from build123d import *

# Parameters (mm, degrees)
F1_DEPTH = 250
F2_R     = 175
F3_DEPTH = 200


with BuildPart() as f1:
    # F0 (on Front) → F1 (new body)
    with BuildSketch(Plane.XZ):
        with BuildLine():
            Line((400, -800), (400, 0))
            ThreePointArc((400, 0), (0, 400), (-400, 0))
            Line((-400, 0), (-400, -800))
            Line((-400, -800), (-150, -800))
            Line((-150, -800), (-150, -606.184542))
            Line((-150, -606.184542), (150, -606.184542))
            Line((150, -606.184542), (150, -800))
            Line((150, -800), (400, -800))
        make_face()
    extrude(amount=F1_DEPTH)

    # F2 (on face) → F3 (join)
    with BuildSketch(Plane.XZ.offset(250)):
        Circle(F2_R)
    extrude(amount=F3_DEPTH)


solid = f1.part
For this review, take the finished solid that the model builds, in its own axes (mm). A direction names the side the tool comes from. Coordinates: 2 decimals unless noted, no trailing zeros. Order: outer loops, then holes, each group sorted by start corner. A loop starts at its lowest first (then second) coordinate and runs counter-clockwise, first axis right, second up. Notation, with made-up numbers: (56, 56) - (65, 56) arc R16 ccw to (65, 65) - close; hole circle Ø10 at (19, 54.5). An arc over 180 degrees is marked (long way). Answer as CSV lines item,"result". Start each with the question number.
1) Add section B-B (x = 0). State the section outline as (y, z) points, then the cut area to 3 significant figures.
2) Insertion check: P1, Ø2, axis at x = 281, y = -96.5, coming from the +Z side; P2, Ø6, axis at x = 112.5, y = -81.5, coming from the -Z side; P3, Ø3, axis at y = -111, z = 117, coming from the -X side. Each pin has a flat end and moves straight along its axis. Give the tip position at first contact, or say it passes through.
3) Add section A-A (y = -94.5). State the section outline as (x, z) points, then the cut area to 3 significant figures.
4) Add section C-C (z = -262.5). State the section outline as (x, y) points, then the cut area to 3 significant figures.
5) Machinability: for faces 1 (the flat face through (-2, -450, 2)), 2 (the flat face through (150, -123, -702)), 3 (the cylindrical face through (-128.982, -348.6, 118.273)), which of the approach directions +Z, -Z, +X, -X, +Y, -Y give a long, thin tool a straight path to every point of the face, cutting with its end or side? Answer none if there is none.
6) Draft analysis for pull direction X (two halves, no side actions). For faces 4 (the flat face through (400, -123, -406)), 5 (the flat face through (-2, -123, -606.185)), 6 (the cylindrical face through (8.796, -123.25, 399.903)), state which applies: +X half, -X half, draft (parallel to the pull), parting line (faces both ways), or undercut.
7) To check wall thickness, follow line 1 along X through (y, z) = (-34.5, -650.5); line 2 along Y through (x, z) = (-284, -90.5); line 3 along X through (y, z) = (-408.5, 9.5). State the ranges of each line that lie inside material, in increasing order. Write a range as [from, to].
8) Add section D-D (y = -280). State the section outline as (x, z) points, then the cut area to 3 significant figures.
Result:
1,outline,"(-450, -175) - (-250, -175) - (-250, -606.18) - (0, -606.18) - (0, 400) - (-250, 400) - (-250, 175) - (-450, 175) - close"
1,area,"322,000 mm^2"
2,P1,"z = 285.66"
2,P2,"z = -606.18"
2,P3,"x = -382.96"
3,outline,"(-400, -800) - (-150, -800) - (-150, -606.18) - (150, -606.18) - (150, -800) - (400, -800) - (400, 0) arc R400 ccw to (-400, 0) - close"
3,area,"833,000 mm^2"
4,outline,"(-400, -250) - (400, -250) - (400, 0) - (-400, 0) - close"
4,area,"200,000 mm^2"
5,face 1,"+Z, -Z, +X, -X, -Y"
5,face 2,"-Z, +Y, -Y"
5,face 3,"-Y"
6,face 4,"+X half"
6,face 5,"undercut"
6,face 6,"parting line"
7,line 1,"[-400, -150], [150, 400]"
7,line 2,"[-250, 0]"
7,line 3,"[-174.74, 174.74]"
8,outline,"circle Ø350 at (0, 0)"
8,area,"96,200 mm^2"
